```python
from build123d import *

# Parameters (mm, degrees)
SKETCH2_R           = 3.429
BOSS_EXTRUDE1_DEPTH = 12.7


with BuildPart() as part:
    # Sketch2 → Boss-Extrude1 (new body)
    with BuildSketch(Plane.XY):
        with BuildLine():
            Line((-4.490128061, 22.450640303), (-22.450640303, 4.490128061))
            ThreePointArc((-22.450640303, 4.490128061), (-24.310512242, 0), (-22.450640303, -4.490128061))
            Line((-22.450640303, -4.490128061), (-4.490128061, -22.450640303))
            ThreePointArc((-4.490128061, -22.450640303), (0, -24.310512242), (4.490128061, -22.450640303))
            Line((4.490128061, -22.450640303), (22.450640303, -4.490128061))
            ThreePointArc((22.450640303, -4.490128061), (24.310512242, 0), (22.450640303, 4.490128061))
            Line((22.450640303, 4.490128061), (4.490128061, 22.450640303))
            ThreePointArc((4.490128061, 22.450640303), (0, 24.310512242), (-4.490128061, 22.450640303))
        make_face()
        with Locations((0, 15.875)):
            Circle(SKETCH2_R, mode=Mode.SUBTRACT)
        with Locations((15.875, 0)):
            Circle(SKETCH2_R, mode=Mode.SUBTRACT)
        with Locations((0, -15.875)):
            Circle(SKETCH2_R, mode=Mode.SUBTRACT)
        with Locations((-15.875, 0)):
            Circle(SKETCH2_R, mode=Mode.SUBTRACT)
        Polygon((5.184753289, 5.184753289), (-1.897751416, 7.082504705), (-7.082504705, 1.897751416), (-5.184753289, -5.184753289), (1.897751416, -7.082504705), (7.082504705, -1.897751416), align=None, mode=Mode.SUBTRACT)
    extrude(amount=BOSS_EXTRUDE1_DEPTH)


solid = part.part
```
Geometry check sheet. Reference: the model listing, model coordinates, mm. A direction names the side the tool comes from. Give positions to 0.01 mm unless a question says otherwise; leave off trailing zeros. Write each loop counter-clockwise with the first axis right and the second up, starting at its lowest first coordinate (ties: lowest second). Pieces come first, ordered by that corner, then holes. Notation, with made-up numbers: (29, -14.5) - (83, -14.5) arc R21 ccw to (83, 24.5) - close; hole circle Ø1 at (11, 80.5). An arc over 180 degrees is marked (long way). Use a Markdown table: item, result.
Q1. Go/stop test with flat-tipped pins: P1, Ø1.5, axis at y = -16.5, z = 7, coming from the +X side; P2, Ø3, axis at x = -13.5, z = 3, coming from the -Y side; P3, Ø3, axis at y = 10, z = 9, coming from the +X side. Record where each tip stops, or that it passes through.
Computed:
| item | result |
|---|---|
| P1 | stops at x = 11.19 |
| P2 | stops at y = -14.94 |
| P3 | stops at x = 18.44 |
Q2. Section check A-A, the plane x = -14. Enter the section's corners in (y, z), then the cut area to 3 significant figures.
Computed:
| item | result |
|---|---|
| outline | (-12.94, 0) - (-2.87, 0) - (-2.87, 12.7) - (-12.94, 12.7) - close; (2.87, 0) - (12.94, 0) - (12.94, 12.7) - (2.87, 12.7) - close |
| area | 256 mm² |
Q3. Set-up check for faces 1 (the face through (0.07, 24.31, 6.26)), 2 (the face through (4.45, -4.53, 6.26)): record each of +Z, -Z, +X, -X, +Y, -Y from which the full face is reachable in a straight line by a thin tool's end or side.
Computed:
| item | result |
|---|---|
| face 1 | +Z, -Z, +Y |
| face 2 | +Z, -Z |
Q4. Draft check along X on faces 3 (the face through (-0.07, -24.31, 6.26)), 4 (the face through (-0.446, 19.275, 6.261)), 5 (the face through (-13.34, 13.6, 6.26)). Enter one of: pulls with the +X half, pulls with the -X half, needs draft (parallel to the pull), parting line crosses it, or undercut.
Computed:
| item | result |
|---|---|
| face 3 | parting line crosses it |
| face 4 | undercut |
| face 5 | pulls with the -X half |
Q5. Section check C-C, the plane z = 3. Give the number of separate pieces and of enclosed holes in the cut face, then the cut area to 3 significant figures.
Computed:
| item | result |
|---|---|
| separate pieces | 1 |
| enclosed holes | 5 |
| area | 1,130 mm² |
Q6. Section check B-B, the plane y = 0. Enter the section's corners in (x, z).
Computed:
| item | result |
|---|---|
| outline | (-24.31, 0) - (-19.3, 0) - (-19.3, 12.7) - (-24.31, 12.7) - close; (-12.45, 0) - (-6.57, 0) - (-6.57, 12.7) - (-12.45, 12.7) - close; (6.57, 0) - (12.45, 0) - (12.45, 12.7) - (6.57, 12.7) - close; (19.3, 0) - (24.31, 0) - (24.31, 12.7) - (19.3, 12.7) - close |
Q7. Thickness scan on L1, parallel to Y at x = 0, z = 9; L2, parallel to X at y = -2, z = 8.25; L3, parallel to X at y = 1.5, z = 8.5. Record the ranges inside material, lowest first. Write a range as [from, to].
Computed:
| item | result |
|---|---|
| L1 | y = [-24.31, -19.3], [-12.45, -6.57], [6.57, 12.45], [19.3, 24.31] |
| L2 | x = [-23.99, -18.66], [-13.09, -6.04], [6.98, 13.09], [18.66, 23.99] |
| L3 | x = [-24.13, -18.96], [-12.79, -6.98], [6.17, 12.79], [18.96, 24.13] |
